from build123d import *

# Parameters (mm, degrees)
BOSS_EXTRUDE2_DEPTH = 7


# Read off the part's stored shape, not the designer's step: CBORE for M3 SHCS1
with BuildPart() as part:
    # Sketch1 → Boss-Extrude2 (new body)
    with BuildSketch(Plane(origin=(0, 0, 0), x_dir=(1, 0, 0), z_dir=(0, 1, 0))):
        with BuildLine():
            Line((14.65303983, 6.875), (24.036105654, 6.875))
            ThreePointArc((24.036105654, 6.875), (20.468816741, 14.353659506), (14.65303983, 20.255577596))
            Line((14.65303983, 20.255577596), (14.65303983, 6.875))
        make_face()
    extrude(amount=BOSS_EXTRUDE2_DEPTH)

    # CBORE for M3 SHCS1 outline → CBORE for M3 SHCS1 (revolve, cut)
    with BuildSketch(Plane(origin=(18.40303983, 0, -10.625), x_dir=(1, 0, 0), z_dir=(0, 0, 1))):
        Polygon((0, 0), (1.6, 0), (1.6, 2.975), (1.625, 3), (3.25, 3), (3.25, 6.975), (3.275, 7), (0, 7), align=None)
    revolve(axis=Axis((18.40303983, 0, -10.625), (0, 1, 0)), mode=Mode.SUBTRACT)


solid = part.part
Input: part model. Units: mm. Frame: model coordinates. A direction names the side the tool comes from. Round coordinates to 2 decimals unless told otherwise and drop trailing zeros. Loops run counter-clockwise (first coordinate to the right, second up) from the corner with the lowest first, then second, coordinate; pieces in that order, holes last. Notation, with made-up numbers: (85.5, 35.5) -> (98.5, 35.5) arc R15 cw to (98.5, 53.5) -> close; hole circle Ø11 at (-4, 87). An arc over 180 degrees is marked (long way). Answer as a JSON object with one key per item and string values. Group by question number.
1) Draft query along Z for faces 1 (the flat face through (19, 3, -6.875)), 2 (the cylindrical face through (19.929, 1.508, -11.106)), 3 (the flat face through (17, 7, -14)). Return one class per face: +Z half, -Z half, draft (parallel to the pull), parting line (faces both ways), or undercut.
2) Section query A-A on y = 3.5. Output: boundary loops of the cut face in (x, z) (3 decimals), plus the area to 3 significant figures.
3) Pin query (flat end, axial travel): pin 1 (4 mm diameter, centred on y = 1, z = -15, fed in from +X). Return the tip coordinate at first contact, or that it passes through.
4) Section query D-D on y = 1. Output: boundary loops of the cut face in (x, z) (3 decimals), plus the area to 3 significant figures.
5) Section query C-C on z = -19.5. Output: boundary loops of the cut face in (x, y).
6) Reachability of faces 4 (the cylindrical face through (21.503, 5.015, -11.601)), 5 (the cylindrical face through (20.536, 3.451, -14.258)) from +Z, -Z, +X, -X, +Y, -Y: full face, straight path, thin tool, end or side. Return the list, or none.
7) Section query B-B on x = 22. Output: boundary loops of the cut face in (y, z) (3 decimals), plus the area to 3 significant figures.
8) Ray query, L1, parallel to Z at x = 15.5, y = 3.75 (3 decimals); L2, parallel to X at y = 2.5, z = -15; L3, parallel to Z at x = 19.75, y = 3.5 (3 decimals). Return the intervals inside material, ascending.
Reply:
{
 "1": {"face 1": "+Z half", "face 2": "undercut", "face 3": "draft"},
 "2": {"outline": "(14.653, -20.256) arc R25 ccw to (24.036, -6.875) -> (14.653, -6.875) -> close; hole circle Ø6.5 at (18.403, -10.625)", "area": "44.6 mm2"},
 "3": {"pin 1": "stops at x = 21.35"},
 "4": {"outline": "(14.653, -20.256) arc R25 ccw to (24.036, -6.875) -> (14.653, -6.875) -> close; hole circle Ø3.2 at (18.403, -10.625)", "area": "69.8 mm2"},
 "5": {"outline": "(14.65, 0) -> (15.64, 0) -> (15.64, 7) -> (14.65, 7) -> close"},
 "6": {"face 4": "+Y", "face 5": "-Z, +X, +Y, -Y"},
 "7": {"outline": "(0, -11.874) -> (7, -11.874) -> (7, -6.875) -> (0, -6.875) -> close", "area": "35.0 mm2"},
 "8": {"L1": "z = -19.615 to -12.086, -9.164 to -6.875", "L2": "x = 14.65 to 20", "L3": "z = -15.328 to -13.583, -7.667 to -6.875"}
}
